```python
from build123d import *

# Parameters (mm, degrees)
BOSS_EXTRUDE1_DEPTH     = 50
SKETCH2_R               = 1.5
BOSS_EXTRUDE2_DEPTH     = 5
SKETCH3_W               = 5
SKETCH3_H               = 1.5
CUT_EXTRUDE1_DEPTH      = 58.879184514
CUT_EXTRUDE1_DEPTH_BACK = 58.879184514
SKETCH4_W               = 45
SKETCH4_H               = 15
BOSS_EXTRUDE3_DEPTH     = 3
SKETCH5_W               = 45
SKETCH5_H               = 15
BOSS_EXTRUDE4_DEPTH     = 3
SKETCH6_R               = 1.5
CUT_EXTRUDE2_DEPTH      = 69.92024376
CUT_EXTRUDE2_DEPTH_BACK = 69.92024376
SKETCH8_W               = 30
SKETCH8_H               = 50
SKETCH8_W_2             = 25
SKETCH8_H_2             = 10
BOSS_EXTRUDE7_DEPTH     = 3
SERVO_MOUNT_DEPTH       = 3


with BuildPart() as part:
    # Sketch1 → Boss-Extrude1 (new body)
    with BuildSketch(Plane.XY):
        Polygon((0, 0), (25, 0), (25, 3), (3, 3), (3, 15), (0, 15), align=None)
    extrude(amount=BOSS_EXTRUDE1_DEPTH)

    # Sketch2 → Boss-Extrude2 (add)
    with BuildSketch(Plane(origin=(0, 3, 0), x_dir=(1, 0, 0), z_dir=(0, 1, 0))):
        with Locations((20, -15)):
            Circle(SKETCH2_R)
        with Locations((20, -35)):
            Circle(SKETCH2_R)
    extrude(amount=BOSS_EXTRUDE2_DEPTH)

    # Sketch3 → Cut-Extrude1 (cut, two sides)
    with BuildSketch(Plane.ZY) as cut_extrude1_sk:
        with Locations((25, 5.25)):
            Rectangle(SKETCH3_W, SKETCH3_H)
    extrude(amount=CUT_EXTRUDE1_DEPTH, mode=Mode.SUBTRACT)
    extrude(cut_extrude1_sk.sketch, amount=-CUT_EXTRUDE1_DEPTH_BACK, mode=Mode.SUBTRACT)

    # Sketch4 → Boss-Extrude3 (add)
    with BuildSketch(Plane(origin=(0, 0, 0), x_dir=(-1, 0, 0), z_dir=(0, 0, -1))):
        with Locations((22.5, 7.5)):
            Rectangle(SKETCH4_W, SKETCH4_H)
    extrude(amount=-BOSS_EXTRUDE3_DEPTH)

    # Sketch5 → Boss-Extrude4 (add)
    with BuildSketch(Plane.XY.offset(50)):
        with Locations((-22.5, 7.5)):
            Rectangle(SKETCH5_W, SKETCH5_H)
    extrude(amount=-BOSS_EXTRUDE4_DEPTH)

    # Sketch6 → Cut-Extrude2 (cut, two sides)
    with BuildSketch(Plane.XY.offset(50)) as cut_extrude2_sk:
        with Locations((-35, 12.5)):
            Circle(SKETCH6_R)
        with Locations((-35, 2.5)):
            Circle(SKETCH6_R)
    extrude(amount=CUT_EXTRUDE2_DEPTH, mode=Mode.SUBTRACT)
    extrude(cut_extrude2_sk.sketch, amount=-CUT_EXTRUDE2_DEPTH_BACK, mode=Mode.SUBTRACT)

    # Sketch8 → Boss-Extrude7 (add)
    with BuildSketch(Plane(origin=(0, 15, 0), x_dir=(1, 0, 0), z_dir=(0, 1, 0))):
        with Locations((-12, -25)):
            Rectangle(SKETCH8_W, SKETCH8_H)
        with Locations((-12, -40)):
            Rectangle(SKETCH8_W_2, SKETCH8_H_2, mode=Mode.SUBTRACT)
    extrude(amount=BOSS_EXTRUDE7_DEPTH)

    # 3DSketch1 → servo mount (add)
    with BuildSketch(Plane(origin=(-27, 18, 30), x_dir=(0.8320502943378437, 0.5547001962252291, 0), z_dir=(0, 0, -1))):
        Polygon((0, 0), (24.96150883, 16.641005887), (36.055512755, 0), (11.094003925, -16.641005887), align=None)
        Polygon((11.78737917, -11.371354023), (30.92453594, 1.386750491), (24.268133585, 11.371354023), (5.130976815, -1.386750491), align=None, mode=Mode.SUBTRACT)
    extrude(amount=SERVO_MOUNT_DEPTH)


solid = part.part
```
Build history of the part. All positions in model axes, mm. A direction names the side the tool comes from. Round coordinates to 2 decimals unless told otherwise and drop trailing zeros. Write each loop counter-clockwise with the first axis right and the second up, starting at its lowest first coordinate (ties: lowest second). Pieces come first, ordered by that corner, then holes. Notation, with made-up numbers: (78, -37) -> (111, -37) arc R23 cw to (111, 2) -> close; hole circle Ø4 at (25.5, -19.5). An arc over 180 degrees is marked (long way). Put each result on its own line as item: value.
Item 1: Slice it at B-B, the plane x = -12.5. Give the cut face in (y, z).
Here are the results:
outline: (0, 0) -> (18, 0) -> (18, 27) -> (22, 27) -> (22, 30) -> (18, 30) -> (18, 35) -> (15, 35) -> (15, 3) -> (0, 3) -> close; (0, 47) -> (15, 47) -> (15, 45) -> (18, 45) -> (18, 50) -> (0, 50) -> close; (34, 27) -> (38, 27) -> (38, 30) -> (34, 30) -> close
Item 2: Flat gauge pins, fed straight in: P1, Ø1, axis at y = 19, z = 22.5, coming from the -X side; P2, Ø24, axis at x = 17.5, z = 36, coming from the +Y side; P3, Ø3.5, axis at y = 25.5, z = 28, coming from the +X side; P4, Ø0.6, axis at x = 0.5, z = 42, coming from the +Y side. Where does each tip first touch, or does it go through?
Here are the results:
P1: passes through
P2: stops at y = 8
P3: stops at x = 3
P4: stops at y = 18
Item 3: Tool access for faces 1 (the face through (1, 4.5, 25)), 2 (the face through (-12, 18, 13)), 3 (the face through (20, 8, 35)): list every direction of +Z, -Z, +X, -X, +Y, -Y with a clear straight run to the whole face (end or side of a thin tool).
Here are the results:
face 1: +X, -X
face 2: -Z, +X, -X, +Y
face 3: +Z, -Z, +X, +Y
Item 4: Slice it at C-C, the plane y = 12.5. Give the cut face in (x, z), plus the area to 3 significant figures.
Here are the results:
outline: (-45, 0) -> (-36.5, 0) -> (-36.5, 3) -> (-45, 3) -> close; (-45, 47) -> (-36.5, 47) -> (-36.5, 50) -> (-45, 50) -> close; (-33.5, 0) -> (3, 0) -> (3, 50) -> (-33.5, 50) -> (-33.5, 47) -> (0, 47) -> (0, 3) -> (-33.5, 3) -> close
area: 402 mm^2
Item 5: Wall check: probe 1 along Y at (x, z) = (-35, 2); probe 2 along Y at (x, z) = (-7.5, 7); probe 3 along X at (y, z) = (2.5, 39.5). Give the ranges that are in metal, low to high. Write a range as from..to.
Here are the results:
probe 1: y = 0..1, 4..11, 14..15
probe 2: y = 15..18
probe 3: x = 0..25
Item 6: Slice it at D-D, the plane x = -35. Give the cut face in (y, z).
Here are the results:
outline: (0, 0) -> (1, 0) -> (1, 3) -> (0, 3) -> close; (0, 47) -> (1, 47) -> (1, 50) -> (0, 50) -> close; (4, 0) -> (11, 0) -> (11, 3) -> (4, 3) -> close; (4, 47) -> (11, 47) -> (11, 50) -> (4, 50) -> close; (14, 0) -> (15, 0) -> (15, 3) -> (14, 3) -> close; (14, 47) -> (15, 47) -> (15, 50) -> (14, 50) -> close
Item 7: Two-plate mould, pull along X, no slides. Class faces 4 (the face through (-11, 21, 27)), 5 (the face through (-45, 7, 1)), 6 (the face through (-36.2, 1.6, 1.5)), 7 (the face through (25, 1, 25)): pulls with the +X half, pulls with the -X half, needs draft (parallel to the pull), parting line crosses it, or undercut.
Here are the results:
face 4: needs draft
face 5: pulls with the -X half
face 6: undercut
face 7: pulls with the +X half
Item 8: Slice it at A-A, the plane z = 43. Give the cut face in (x, y), plus the area to 3 significant figures.
Here are the results:
outline: (-27, 15) -> (-24.5, 15) -> (-24.5, 18) -> (-27, 18) -> close; (0, 0) -> (25, 0) -> (25, 3) -> (3, 3) -> (3, 18) -> (0.5, 18) -> (0.5, 15) -> (0, 15) -> close
area: 126 mm^2
